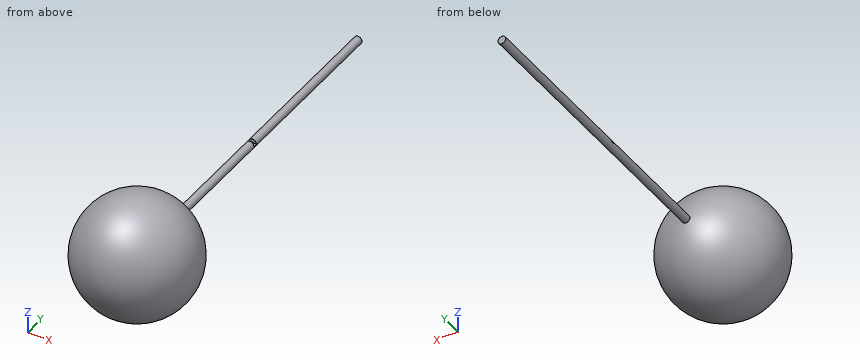
from build123d import *

# Parameters (mm, degrees)
CROQUIS3_R                 = 1
SALIENTE_EXTRUIR1_DEPTH    = 90
CORTAR_EXTRUIR1_DEPTH      = 10
CORTAR_EXTRUIR1_DEPTH_BACK = 10
CROQUIS4_W                 = 4.139739446
CROQUIS4_H                 = 1


with BuildPart() as part:
    # Croquis2 → Revoluci_n1 (revolve)
    with BuildSketch(Plane.XY):
        with BuildLine():
            Line((0, 15), (0, 13.292119178))
            ThreePointArc((0, 13.292119178), (-13.292119178, 0), (0, -13.292119178))
            Line((0, -13.292119178), (0, -15))
            ThreePointArc((0, -15), (-15, 0), (0, 15))
        make_face()
    revolve(axis=Axis((0, 15, 0), (0, -1, 0)))

    # Croquis3 → Saliente-Extruir1 (add)
    with BuildSketch(Plane(origin=(0, 0, 0), x_dir=(1, 0, 0), z_dir=(0, 1, 0))):
        with Locations(Location((0, 0, 0), (0, 0, 90))):
            Circle(CROQUIS3_R)
    extrude(amount=SALIENTE_EXTRUIR1_DEPTH)

    # Croquis4 → Cortar-Extruir1 (cut, two sides: drawn at the far end of the back side and taken through both)
    with BuildSketch(Plane(origin=(0, 0, 0), x_dir=(0, 0, -1), z_dir=(1, 0, 0)).offset(-CORTAR_EXTRUIR1_DEPTH_BACK)):
        with Locations((-2.069869723, 46.5)):
            Rectangle(CROQUIS4_W, CROQUIS4_H)
    extrude(amount=CORTAR_EXTRUIR1_DEPTH + CORTAR_EXTRUIR1_DEPTH_BACK, mode=Mode.SUBTRACT)


solid = part.part
Geometry check sheet. Reference: the model listing, model coordinates, mm. Give positions to 0.01 mm unless a question says otherwise; leave off trailing zeros. Order: outer loops, then holes, each group sorted by start corner. A loop starts at its lowest first (then second) coordinate and runs counter-clockwise, first axis right, second up. Notation, with made-up numbers: (-31.75, 17.25) - (1.25, 17.25) arc R18 ccw to (1.25, 41.25) - close; hole circle Ø2 at (37.25, -9). An arc over 180 degrees is marked (long way). Use one line per item in the form item = value.
1) Sectioned sample at A-A (x = 0). Record the boundary of the cut face in (y, z).
Working result:
outline = (14.97, -1) - (90, -1) - (90, 1) - (47, 1) - (47, 0) - (46, 0) - (46, 1) - (14.97, 1) arc R15 ccw (long way) to start; hole (0, -1) - (0, 1) - (13.25, 1) arc R13.29 ccw (long way) to (13.25, -1) - close
2) Sectioned sample at D-D (y = 57). Record the boundary of the cut face in (x, z), and give its area (3 significant figures).
Working result:
outline = circle Ø2 at (0, 0)
area = 3.14 mm^2
3) Depth check by flat-ended pin: pin 1 Ø1 at (x, z) = (8.5, -10) entering from +Y; pin 2 Ø8 at (x, z) = (-8.5, 10.5) entering from +Y; pin 3 Ø10 at (x, y) = (-3, 58.5) entering from +Z. Enter the tip coordinate at first touch or a pass-through.
Working result:
pin_1 = 8.1
pin_2 = 11.6
pin_3 = 1
4) Material ranges on probe 1 along Y at (x, z) = (-0.25, 0.25); probe 2 along Y at (x, z) = (-8.25, -2.25); probe 3 along Y at (x, z) = (1.5, -0.5), recorded low to high. Write a range as from..to.
Working result:
probe_1 = -15..-13.29, 0..46, 47..90
probe_2 = -12.32..-10.18, 10.18..12.32
probe_3 = -14.92..-13.2, 13.2..14.92
5) Sectioned sample at C-C (z = 4.25). Record the boundary of the cut face in (x, y).
Working result:
outline = circle Ø28.77 at (0, 0); hole circle Ø25.19 at (0, 0)
6) Sectioned sample at B-B (y = 8). Record the boundary of the cut face in (x, z), and give its area (3 significant figures).
Working result:
outline = circle Ø25.38 at (0, 0); circle Ø2 at (0, 0); hole circle Ø21.23 at (0, 0)
area = 155 mm^2
